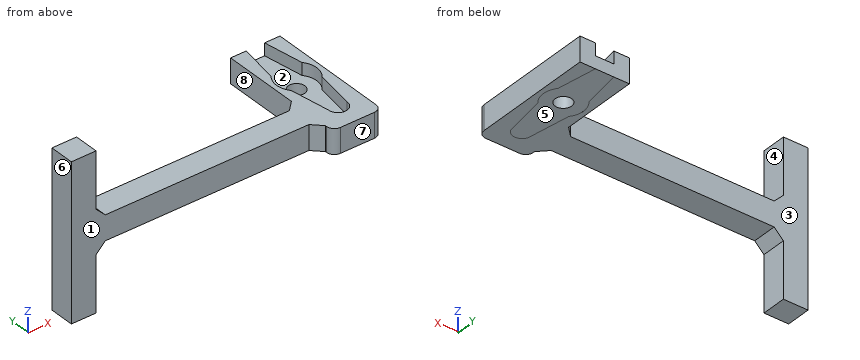
Autodesk Inventor part; units mm, degrees
ref_plane "YZ Plane" through (0, 0, 0) normal (1, 0, 0) x (0, 1, 0)
ref_plane "XZ Plane" through (0, 0, 0) normal (0, 1, 0) x (-1, 0, 0)
ref_plane "XY Plane" through (0, 0, 0) normal (0, 0, 1) x (1, 0, 0)
sketch "Skizze2" plane through (0, 0, 0) normal (0, 0, 1) x (1, 0, 0)
  line L0 (-19.9249, 0) -> (3.9249, 0)
  line L1 (0, -18.1036) -> (0, 108.6213)
  circle A0 centre (-8, 65) radius 2.7
  line L2 (0, 0) -> (0, 87.5)
  arc A1 (0, 87.5) -> (-2.5, 90) centre (-2.5, 87.5) ccw
  line L3 (-13.5, 90) -> (-2.5, 90)
  arc A2 (-13.5, 90) -> (-16, 87.5) centre (-13.5, 87.5) ccw
  line L4 (0, 42.5) -> (0, 87.5)
  line L5 (-16, 40) -> (-16, 87.5)
  line L6 (0, 40) -> (-16, 40)
  point P0 (-8, 90)
  dimension "d4" = 2.5
  dimension "d5" = 2.5
  dimension "d6" = 5.4
  dimension "d8" = 25
  dimension "d17" = 2.5
  dimension "d18" = 2.5
  dimension "d19" = 2.5
  dimension "d144" = 25
extrude "Extrusion1" add sketch "Skizze2" along normal mid plane 8
sketch "Skizze7" plane through (0, 0, -4) normal (0, 0, -1) x (-1, 0, 0)
  arc A0 (16, 87.5) -> (13.5, 90) centre (13.5, 87.5) ccw
  line L0 (13.5, 90) -> (2.5, 90)
  arc A1 (2.5, 90) -> (0, 87.5) centre (2.5, 87.5) ccw
  line L1 (0, 87.5) -> (0, 40)
  circle A2 centre (8, 65) radius 2.7
  circle A3 centre (8, 65) radius 6.5
  line L2 (8, 85) -> (8, 45)
  line L3 (13, 82.2483) -> (13, 48.2483)
  line L4 (3, 48.3648) -> (3, 82.3648)
  line L5 (16, 40) -> (16, 87.5)
  line L6 (0, 40) -> (16, 40)
  circle A4 centre (8, 82) radius 3
  circle A5 centre (8, 48) radius 3
  line L7 (-2, 82) -> (18, 82)
  line L8 (-2, 48) -> (18, 48)
  line L9 (5, 48) -> (3, 60.8467)
  line L10 (11, 48) -> (13, 60.8467)
  line L11 (3, 69.1533) -> (5, 82)
  line L12 (13, 69.1533) -> (11, 82)
  point P0 (0, 0)
  point P1 (8, 65)
  dimension "d133" = 13
  dimension "d136" = 20
  dimension "d137" = 20
  dimension "d194" = 6
  dimension "d195" = 6
  dimension "d196" = 3
  dimension "d197" = 3
  dimension "d198" = 10
  dimension "d199" = 20
  dimension "d200" = 20
extrude "Extrusion5" cut sketch "Skizze7" against normal blind 0.001 contours L8 L2 A5 | A5 L2 L8 | A5 L2 A3 L10 | L3 A3 L2 A2 | A3 L3 | A3 L2 A4 L12 | L7 L2 A4 | A4 L2 L7 | A5 L8 L2 | A5 L9 A3 L2 | L2 L8 A5 | L2 A2 A3 L4 | A3 L11 A4 L2 | L2 L7 A4 | A4 L7 L2 | L4 A3
fillet "Rundung2" radius 2.5 2 edges at (0, 40, 0) (-16, 40, 0)
sketch "Skizze12" plane through (-16, 40, 4) normal (-1, 0, 0) x (0, 0, 1)
  line L0 (0, 47.5) -> (0, 0)
  line L1 (-8, 0) -> (-8, 47.5)
  line L2 (0, 47.5) -> (0, 2.5)
  line L3 (-8, 47.5) -> (0, 47.5)
  line L4 (-8, 2.5) -> (-8, 47.5)
  line L5 (0, 6) -> (-8, 6)
  line L6 (-8, 6) -> (-8, 14)
  line L7 (-8, 14) -> (0, 14)
  line L8 (0, 14) -> (0, 6)
  line L9 (0, 2.5) -> (-8, 2.5)
  point P0 (-4, -40)
  point P1 (0, 8)
  point P2 (-4, 20.6699)
  point P3 (0, 14)
  dimension "d184" = 8
extrude "Extrusion10" add sketch "Skizze12" along normal blind 80 contours L0 L5 L1 L7
sketch "Skizze17" plane through (-16, 54, 4) normal (0, 1, 0) x (1, 0, 0)
  line L0 (-80, 0) -> (-80, 8)
  line L1 (-72, 29) -> (-80, 29)
  line L2 (-72, -21) -> (-80, -21)
  line L3 (-80, 29) -> (-80, -21)
  line L4 (-72, 29) -> (-72, -21)
  line L5 (0, 8) -> (0, 0)
  line L6 (0, 8) -> (-80, 8)
  line L7 (-80, 0) -> (-80, 8)
  line L8 (0, 0) -> (-80, 0)
  line L9 (-80, 4) -> (0, 4)
  point P0 (16, 4)
  point P1 (-80, 8)
  dimension "d187" = 50
  dimension "d188" = 8
extrude "Extrusion15" add sketch "Skizze17" against normal blind 8 contours L8 L4 L2 L3 | L0 L9 L4 L8 | L0 L6 L4 L9 | L3 L1 L4 L6
chamfer "Fasen10" distance 3 angle 45 4 edges at (-16, 46, 0) (-16, 54, 0) (-88, 50, -4) (-88, 50, 4)
sketch "Skizze18" plane through (0, 0, 4) normal (0, 0, 1) x (1, 0, 0)
  circle A0 centre (-8, 65) radius 2.7
  arc A1 (-13, 69.1533) -> (-13, 60.8467) centre (-8, 65) ccw
  line L0 (-11, 82) -> (-13, 69.1533)
  arc A2 (-5, 82) -> (-11, 82) centre (-8, 82) ccw
  line L1 (-3, 69.1533) -> (-5, 82)
  arc A3 (-3, 60.8467) -> (-3, 69.1533) centre (-8, 65) ccw
  line L2 (-5, 48) -> (-3, 60.8467)
  arc A4 (-11, 48) -> (-5, 48) centre (-8, 48) ccw
  line L3 (-13, 60.8467) -> (-11, 48)
  circle A5 centre (-8, 65) radius 2.7
  point P0 (0, 0)
extrude "Extrusion16" cut sketch "Skizze18" against normal blind 4
sketch "Skizze19" plane through (-13.5, 90, 4) normal (0, 1, 0) x (1, 0, 0)
  line L0 (11, 0) -> (0, 0)
  line L1 (0, 8) -> (11, 8)
  line L2 (11, 8) -> (11, 0)
  line L3 (13.5, 0) -> (11, 0)
  line L4 (13.5, 8) -> (13.5, 0)
  line L5 (11, 8) -> (13.5, 8)
  line L6 (-2.5, 8) -> (-2.5, 0)
  line L7 (0, 0) -> (-2.5, 0)
  line L8 (0, 0) -> (0, 8)
  line L9 (-2.5, 8) -> (0, 8)
  point P0 (13.5, 4)
extrude "Extrusion17" cut sketch "Skizze19" against normal blind 8
properties part number "Gripper neu"
Part model, mm, in its own coordinate system. Face numbers are marked on the shaded views. A direction names the side the tool comes from. Round coordinates to 2 decimals unless told otherwise and drop trailing zeros. Write each loop counter-clockwise with the first axis right and the second up, starting at its lowest first coordinate (ties: lowest second). Pieces come first, ordered by that corner, then holes. Notation, with made-up numbers: M 38,32.5 L 97,32.5 A21 cw 97,47.5 Z; hole C 40.25,78 d4. An arc over 180 degrees is marked long. Answer as CSV lines item,"result". Start each with the question number.
1) Drop flat-ended pins along their axis: pin 1 (15 mm diameter, centred on x = -49.5, z = -0.5, fed in from -Y); pin 2 (7 mm diameter, centred on x = -8, y = 65, fed in from -Z); pin 3 (10 mm diameter, centred on x = -64, y = 53, fed in from +Z); pin 4 (5 mm diameter, centred on x = -16, z = 8, fed in from -Y). Give the stop position or say it passes through.
2) Which spindle directions (+Z, -Z, +X, -X, +Y, -Y) get a long thin tool onto all of the face, cutting with end or side? Do the marked faces 4, 5, 6, 7 and 8. Say none if no direction does.
3) Mould opens along Y. For the marked faces 1, 2 and 3 say: +Y half, -Y half, draft (parallel to the pull), parting line (faces both ways), or undercut.
4) Band-saw the part on A-A (z = -1). List the corners of the cut face in (x, y), then the cut area to 3 significant figures.
5) Drill centre lines: L1, parallel to X at y = 65, z = -2.05; L2, parallel to Y at x = -8, z = -2; L3, parallel to Z at x = -58, y = 50. Where is each one in solid material? Low to high.
Worked out:
1,pin 1,"y = 46"
1,pin 2,"z = -4"
1,pin 3,"z = 4"
1,pin 4,"through"
2,face 4,"+Z, +X, +Y, -Y"
2,face 5,"-Z, +X, +Y, -Y"
2,face 6,"+Z, -Z, -X, +Y, -Y"
2,face 7,"+Z, -Z, +X, -X, -Y"
2,face 8,"+Z, -Z, -X, +Y"
3,face 1,"-Y half"
3,face 2,"undercut"
3,face 3,"+Y half"
4,outline,"M -96,46 L -19,46 L -16,43 L -16,42.5 A2.5 ccw -13.5,40 L -2.5,40 A2.5 ccw 0,42.5 L 0,82 L -16,82 L -16,57 L -19,54 L -96,54 Z; hole C -8,65 d5.4"
4,area,"1,300 mm²"
5,L1,"-16 to -10.7, -5.3 to 0"
5,L2,"40 to 62.3, 67.7 to 82"
5,L3,"-4 to 4"
